Model file for the job. Use its own axes, mm. Face numbers are marked on the shaded views. A direction names the side the tool comes from. Round coordinates to 2 decimals unless told otherwise and drop trailing zeros. Loops run counter-clockwise (first coordinate to the right, second up) from the corner with the lowest first, then second, coordinate; pieces in that order, holes last. Notation, with made-up numbers: (40, -20) -> (96, -20) arc R32 cw to (96, 8) -> close; hole circle Ø5 at (76, -12.75). An arc over 180 degrees is marked (long way). Use a Markdown table: item, result.
from build123d import *

# Parameters (mm, degrees)
BOSS_EXTRUDE1_DEPTH = 3.175
SKETCH2_R           = 4.7625
BOSS_EXTRUDE2_DEPTH = 2.032
CUT_EXTRUDE1_DEPTH  = 17.018


with BuildPart() as part:
    # Sketch1 → Boss-Extrude1 (new body)
    with BuildSketch(Plane.XY):
        with BuildLine():
            Line((0, 4.445), (0.515524368, 3.132867636))
            ThreePointArc((0.515524368, 3.132867636), (0.522587824, 3.131697138), (0.529648623, 3.130510715))
            Line((0.529648623, 3.130510715), (1.443289141, 4.204157639))
            Line((1.443289141, 4.204157639), (1.504832294, 2.795729738))
            ThreePointArc((1.504832294, 2.795729738), (1.511132973, 2.79232916), (1.517425967, 2.788914383))
            Line((1.517425967, 2.788914383), (2.730175508, 3.507729564))
            Line((2.730175508, 3.507729564), (2.331068291, 2.155631142))
            ThreePointArc((2.331068291, 2.155631142), (2.335923416, 2.15036899), (2.340766663, 2.145095903))
            Line((2.340766663, 2.145095903), (3.721204996, 2.431184563))
            Line((3.721204996, 2.431184563), (2.904696869, 1.281936464))
            ThreePointArc((2.904696869, 1.281936464), (2.907580312, 1.275382973), (2.910448969, 1.268822997))
            Line((2.910448969, 1.268822997), (4.308984182, 1.09118299))
            Line((4.308984182, 1.09118299), (3.16355647, 0.269324079))
            ThreePointArc((3.16355647, 0.269324079), (3.164155765, 0.262189422), (3.16473897, 0.255053432))
            Line((3.16473897, 0.255053432), (4.429818071, -0.367065191))
            Line((4.429818071, -0.367065191), (3.07959564, -0.772473749))
            ThreePointArc((3.07959564, -0.772473749), (3.077845844, -0.779416422), (3.076080397, -0.78635513))
            Line((3.076080397, -0.78635513), (4.070612437, -1.785536163))
            Line((4.070612437, -1.785536163), (2.661912838, -1.730562061))
            ThreePointArc((2.661912838, -1.730562061), (2.658003568, -1.736560402), (2.654080783, -1.742549913))
            Line((2.654080783, -1.742549913), (3.270292783, -3.010516586))
            Line((3.270292783, -3.010516586), (1.955770475, -2.50111712))
            ThreePointArc((1.955770475, -2.50111712), (1.950125363, -2.505521117), (1.944470334, -2.509912373))
            Line((1.944470334, -2.509912373), (2.115586162, -3.909260824))
            Line((2.115586162, -3.909260824), (1.037690035, -3.000637331))
            ThreePointArc((1.037690035, -3.000637331), (1.030920815, -3.002969742), (1.024146352, -3.005286883))
            Line((1.024146352, -3.005286883), (0.731622954, -4.384375994))
            Line((0.731622954, -4.384375994), (0.007159778, -3.174991927))
            ThreePointArc((0.007159778, -3.174991927), (0, -3.175), (-0.007159778, -3.174991927))
            Line((-0.007159778, -3.174991927), (-0.731622954, -4.384375994))
            Line((-0.731622954, -4.384375994), (-1.024146352, -3.005286883))
            ThreePointArc((-1.024146352, -3.005286883), (-1.030920815, -3.002969742), (-1.037690035, -3.000637331))
            Line((-1.037690035, -3.000637331), (-2.115586162, -3.909260824))
            Line((-2.115586162, -3.909260824), (-1.944470334, -2.509912373))
            ThreePointArc((-1.944470334, -2.509912373), (-1.950125363, -2.505521117), (-1.955770475, -2.50111712))
            Line((-1.955770475, -2.50111712), (-3.270292783, -3.010516586))
            Line((-3.270292783, -3.010516586), (-2.654080783, -1.742549913))
            ThreePointArc((-2.654080783, -1.742549913), (-2.658003568, -1.736560402), (-2.661912838, -1.730562061))
            Line((-2.661912838, -1.730562061), (-4.070612437, -1.785536163))
            Line((-4.070612437, -1.785536163), (-3.076080397, -0.78635513))
            ThreePointArc((-3.076080397, -0.78635513), (-3.077845844, -0.779416422), (-3.07959564, -0.772473749))
            Line((-3.07959564, -0.772473749), (-4.429818071, -0.367065191))
            Line((-4.429818071, -0.367065191), (-3.16473897, 0.255053432))
            ThreePointArc((-3.16473897, 0.255053432), (-3.164155765, 0.262189422), (-3.16355647, 0.269324079))
            Line((-3.16355647, 0.269324079), (-4.308984182, 1.09118299))
            Line((-4.308984182, 1.09118299), (-2.910448969, 1.268822997))
            ThreePointArc((-2.910448969, 1.268822997), (-2.907580312, 1.275382973), (-2.904696869, 1.281936464))
            Line((-2.904696869, 1.281936464), (-3.721204996, 2.431184563))
            Line((-3.721204996, 2.431184563), (-2.340766663, 2.145095903))
            ThreePointArc((-2.340766663, 2.145095903), (-2.335923416, 2.15036899), (-2.331068291, 2.155631142))
            Line((-2.331068291, 2.155631142), (-2.730175508, 3.507729564))
            Line((-2.730175508, 3.507729564), (-1.517425967, 2.788914383))
            ThreePointArc((-1.517425967, 2.788914383), (-1.511132973, 2.79232916), (-1.504832294, 2.795729738))
            Line((-1.504832294, 2.795729738), (-1.443289141, 4.204157639))
            Line((-1.443289141, 4.204157639), (-0.529648623, 3.130510715))
            ThreePointArc((-0.529648623, 3.130510715), (-0.522587824, 3.131697138), (-0.515524368, 3.132867636))
            Line((-0.515524368, 3.132867636), (0, 4.445))
        make_face()
    extrude(amount=BOSS_EXTRUDE1_DEPTH)

    # Sketch2 → Boss-Extrude2 (add)
    with BuildSketch(Plane(origin=(0, 0, 0), x_dir=(-1, 0, 0), z_dir=(0, 0, -1))):
        Circle(SKETCH2_R)
    extrude(amount=BOSS_EXTRUDE2_DEPTH)

    # Mirror1: part across plane


with BuildPart() as part_1:
    add(part.part)
    add(part.part.mirror(Plane.XY.offset(3.175)))

    # Sketch3 → Cut-Extrude1 (cut)
    with BuildSketch(Plane(origin=(0, 0, -2.032), x_dir=(-1, 0, 0), z_dir=(0, 0, -1))):
        with BuildLine():
            Line((-0.635, 2.418010546), (-0.635, 1.484))
            Line((-0.635, 1.484), (0.635, 1.484))
            Line((0.635, 1.484), (0.635, 2.418010546))
            ThreePointArc((0.635, 2.418010546), (0, -2.5), (-0.635, 2.418010546))
        make_face()
    extrude(amount=-CUT_EXTRUDE1_DEPTH, mode=Mode.SUBTRACT)


solid = part_1.part
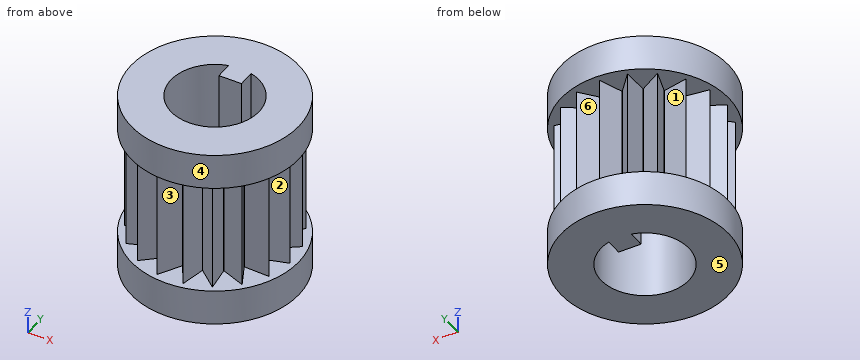
Q1. Pull direction X, two halves, no side cores. Call the marked faces 4, 5 and 6: released by +X, released by -X, zero draft, split by the parting line, or undercut.
Results list:
| item | result |
|---|---|
| face 4 | split by the parting line |
| face 5 | zero draft |
| face 6 | undercut |
Q2. Tool access for the marked faces 1, 2 and 3: list every direction of +Z, -Z, +X, -X, +Y, -Y with a clear straight run to the whole face (end or side of a thin tool).
Results list:
| item | result |
|---|---|
| face 1 | none |
| face 2 | +X |
| face 3 | -Y |
Q3. Drill centre lines: L1, parallel to Z at x = -2.5, y = 3.75; L2, parallel to X at y = 4, z = 0.5; L3, parallel to X at y = 1.75, z = 2 (3 decimals). Where is each one in solid material? Low to high. Write a range as from..to.
Results list:
| item | result |
|---|---|
| L1 | z = -2.03..0, 6.35..8.38 |
| L2 | x = -1.45..-1.27, -0.17..0.17, 1.27..1.45 |
| L3 | x = -3.237..-1.785, -0.635..0.635, 1.785..3.237 |
Q4. Band-saw the part on B-B, the plane z = -0.5. Give the cut face in (x, y) (1 decimal), plus the area to 3 significant figures.
Results list:
| item | result |
|---|---|
| outline | circle Ø9.5 at (0, 0); hole (-0.6, 1.5) -> (-0.6, 2.4) arc R2.5 ccw (long way) to (0.6, 2.4) -> (0.6, 1.5) -> close |
| area | 52.9 mm² |
Q5. Band-saw the part on A-A, the plane y = -1.5. Give the cut face in (x, z).
Results list:
| item | result |
|---|---|
| outline | (-4.52, -2.03) -> (-2, -2.03) -> (-2, 8.38) -> (-4.52, 8.38) -> (-4.52, 6.35) -> (-3.79, 6.35) -> (-3.79, 0) -> (-4.52, 0) -> close; (2, -2.03) -> (4.52, -2.03) -> (4.52, 0) -> (3.79, 0) -> (3.79, 6.35) -> (4.52, 6.35) -> (4.52, 8.38) -> (2, 8.38) -> close |
Q6. Band-saw the part on C-C, the plane x = 3.5. Give the cut face in (y, z), plus the area to 3 significant figures.
Results list:
| item | result |
|---|---|
| outline | (-3.23, -2.03) -> (3.23, -2.03) -> (3.23, 0) -> (2.39, 0) -> (2.39, 6.35) -> (3.23, 6.35) -> (3.23, 8.38) -> (-3.23, 8.38) -> (-3.23, 6.35) -> (-1.76, 6.35) -> (-1.76, 0) -> (-3.23, 0) -> close; hole (-1.21, 0) -> (-0.65, 0) -> (-0.65, 6.35) -> (-1.21, 6.35) -> close; hole (0.09, 0) -> (0.51, 0) -> (0.51, 6.35) -> (0.09, 6.35) -> close; hole (1.19, 0) -> (2.12, 0) -> (2.12, 6.35) -> (1.19, 6.35) -> close |
| area | 40.5 mm² |
Q7. Band-saw the part on D-D, the plane x = 1.75. Give the cut face in (y, z).
Results list:
| item | result |
|---|---|
| outline | (-4.43, -2.03) -> (-1.79, -2.03) -> (-1.79, 8.38) -> (-4.43, 8.38) -> (-4.43, 6.35) -> (-3.6, 6.35) -> (-3.6, 0) -> (-4.43, 0) -> close; (1.79, -2.03) -> (4.43, -2.03) -> (4.43, 0) -> (2.93, 0) -> (2.93, 6.35) -> (4.43, 6.35) -> (4.43, 8.38) -> (1.79, 8.38) -> close |
Q8. Flat gauge pins, fed straight in: pin 1 (0.5 mm diameter, centred on y = 2, z = 3.5, fed in from -X); pin 2 (0.5 mm diameter, centred on y = 2, z = 2.5, fed in from +X); pin 3 (2 mm diameter, centred on y = -3, z = 5, fed in from -X). Where does each tip first touch, or does it go through?
Results list:
| item | result |
|---|---|
| pin 1 | stops at x = -3.59 |
| pin 2 | stops at x = 3.59 |
| pin 3 | stops at x = -3.27 |
